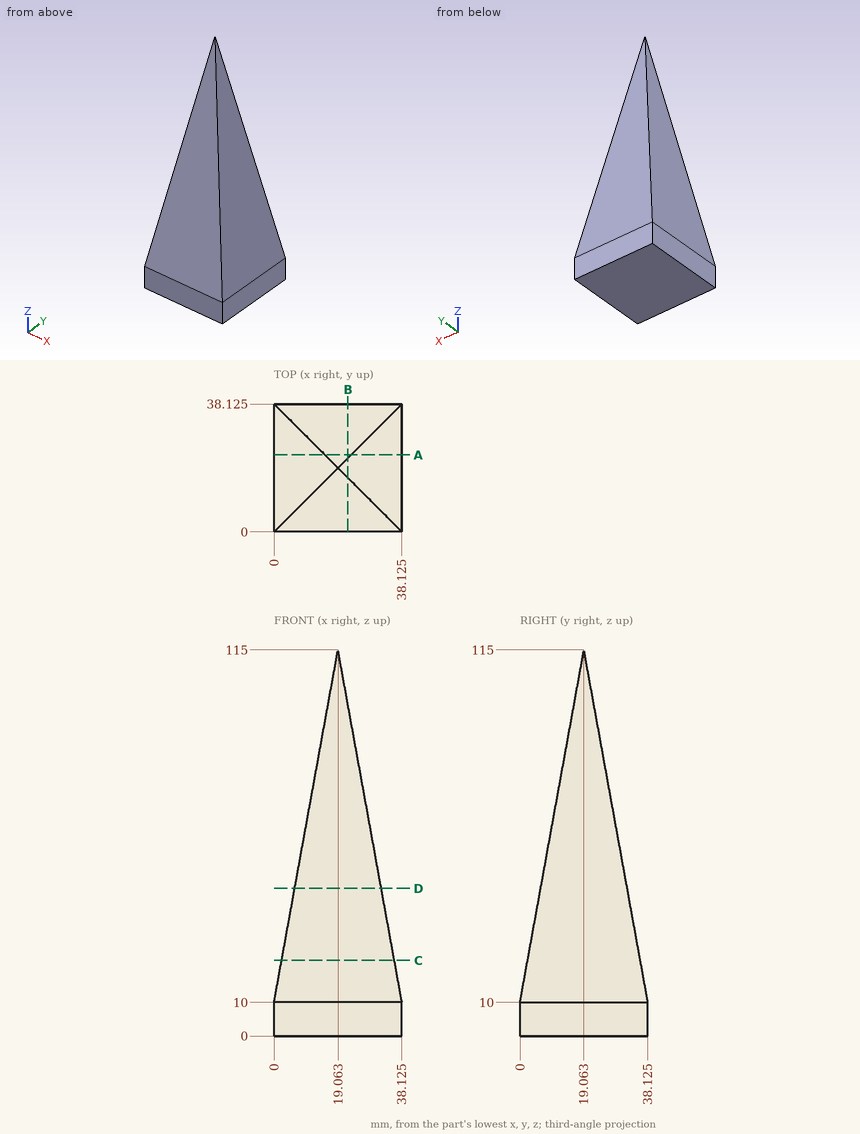
Study the drawing (mm; zero at the part's minimum x, y, z) and answer. Round coordinates to 2 decimals unless told otherwise and drop trailing zeros. Order: outer loops, then holes, each group sorted by start corner. A loop starts at its lowest first (then second) coordinate and runs counter-clockwise, first axis right, second up. Notation, with made-up numbers: (51, -8) -> (71, -8) arc R18 cw to (71, 12) -> close; hole circle Ø2 at (-11, 85). An arc over 180 degrees is marked (long way). Write each question's results on one line, items separated by ' | '. Start each with the question number.
Q1. Find section A-A (y = 23). Determine the outline of the cut face in (x, z) (1 decimal), then the cut area to 3 significant figures.
Q2. Find section D-D (z = 44). Determine the outline of the cut face in (x, y).
Q3. Each of these flat-tipped pins is pushed along its axis until it touches: pin 1 (10 mm diameter, centred on x = 22, y = 8.5, fed in from -Z); pin 2 (8 mm diameter, centred on x = 27.5, z = 33, fed in from +Y) (1 decimal); pin 3 (3 mm diameter, centred on x = 30.5, z = 25, fed in from -Y); pin 4 (1 mm diameter, centred on y = 6, z = 24, fed in from -X). Where does it stop, or does it pass through?
Q4. Find section B-B (x = 22). Determine the outline of the cut face in (y, z) (1 decimal).
Q5. Straight lines are drawn through the part: probe 1 along Y at (x, z) = (22, 22); probe 2 along X at (y, z) = (6.5, 30.5); probe 3 along Y at (x, z) = (33, 30) (1 decimal). For each, find the intervals that lie inside material, in ascending order. Write a range as from..to.
Q6. Find section C-C (z = 22.5). Determine the outline of the cut face in (x, y) (1 decimal), then the cut area to 3 significant figures.
Worked answers:
1) outline: (0, 0) -> (38.1, 0) -> (38.1, 10) -> (23, 93.3) -> (15.1, 93.3) -> (0, 10) -> close | area: 2,300 mm2
2) outline: (6.17, 6.17) -> (31.95, 6.17) -> (31.95, 31.95) -> (6.17, 31.95) -> close
3) pin 1: stops at z = 0 | pin 2: stops at y = 34.7 | pin 3: stops at y = 2.45 | pin 4: stops at x = 2.45
4) outline: (0, 0) -> (38.1, 0) -> (38.1, 10) -> (22, 98.8) -> (16.1, 98.8) -> (0, 10) -> close
5) probe 1: y = 2.18..35.95 | probe 2: x = 3.72..34.4 | probe 3: y = 3.6..34.5
6) outline: (2.3, 2.3) -> (35.9, 2.3) -> (35.9, 35.9) -> (2.3, 35.9) -> close | area: 1,130 mm2
